The listing builds one solid part. Answer for the finished solid, in the listing's coordinates (mm). Give positions to 0.01 mm unless a question says otherwise; leave off trailing zeros. Write each loop counter-clockwise with the first axis right and the second up, starting at its lowest first coordinate (ties: lowest second). Pieces come first, ordered by that corner, then holes. Notation, with made-up numbers: (4.25, 54.25) -> (38.25, 54.25) arc R26 cw to (38.25, 81.25) -> close; hole circle Ø2 at (77.25, -2). An arc over 180 degrees is marked (long way). One line per question, with ' | ' between items.
from build123d import *

# Parameters (mm, degrees)
SKETCH_1_R      = 40
SKETCH_1_R_2    = 3.25
SKETCH_1_R_3    = 8.5
SKETCH_1_R_4    = 2.5
EXTRUDE_1_DEPTH = 4


with BuildPart() as part:
    # 草图1 → 凸台-拉伸1 (new body)
    with BuildSketch(Plane.XY):
        Circle(SKETCH_1_R)
        with Locations((0, 35)):
            Circle(SKETCH_1_R_2, mode=Mode.SUBTRACT)
        with Locations((30.310889132, 17.5)):
            Circle(SKETCH_1_R_2, mode=Mode.SUBTRACT)
        with Locations((30.310889132, -17.5)):
            Circle(SKETCH_1_R_2, mode=Mode.SUBTRACT)
        with Locations((0, -35)):
            Circle(SKETCH_1_R_2, mode=Mode.SUBTRACT)
        with Locations((-30.310889132, -17.5)):
            Circle(SKETCH_1_R_2, mode=Mode.SUBTRACT)
        with Locations((-30.310889132, 17.5)):
            Circle(SKETCH_1_R_2, mode=Mode.SUBTRACT)
        Circle(SKETCH_1_R_3, mode=Mode.SUBTRACT)
        with Locations((-9.25, 16.02146997)):
            Circle(SKETCH_1_R_4, mode=Mode.SUBTRACT)
        with Locations((16.02146997, 9.25)):
            Circle(SKETCH_1_R_4, mode=Mode.SUBTRACT)
        with Locations((9.25, -16.02146997)):
            Circle(SKETCH_1_R_4, mode=Mode.SUBTRACT)
        with Locations((-16.02146997, -9.25)):
            Circle(SKETCH_1_R_4, mode=Mode.SUBTRACT)
    extrude(amount=EXTRUDE_1_DEPTH)


solid = part.part
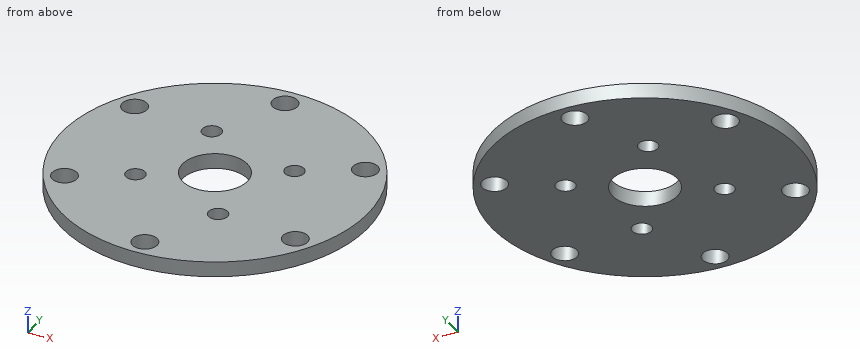
Item 1: Consider line 1 (Y direction, x = 0, z = 2.4); line 2 (Y direction, x = -30, z = 1.6); line 3 (Y direction, x = -2, z = 1.6). Determine where each line is inside the solid, lowest interval first. Write a range as [from, to].
Answers below:
line 1: [-40, -38.25], [-31.75, -8.5], [8.5, 31.75], [38.25, 40] | line 2: [-26.46, -20.74], [-14.26, 14.26], [20.74, 26.46] | line 3: [-39.95, -37.56], [-32.44, -8.26], [8.26, 32.44], [37.56, 39.95]
Item 2: Find section C-C (z = 2.9). Count the separate pieces of the cut face and the enclosed holes in it, then the cut area to 3 significant figures.
Answers below:
separate pieces: 1 | enclosed holes: 11 | area: 4,520 mm²
Item 3: Find section D-D (y = -24). Write down the section's boundary in (x, z), then the cut area to 3 significant figures.
Answers below:
outline: (-32, 0) -> (32, 0) -> (32, 4) -> (-32, 4) -> close | area: 256 mm²
Item 4: Find section A-A (y = 33). Write down the section's boundary in (x, z), then the cut area to 3 significant figures.
Answers below:
outline: (-22.61, 0) -> (-2.56, 0) -> (-2.56, 4) -> (-22.61, 4) -> close; (2.56, 0) -> (22.61, 0) -> (22.61, 4) -> (2.56, 4) -> close | area: 160 mm²
Item 5: Flat-ended cylindrical pins translate along their axes: pin 1 (5 mm diameter, centred on x = 0, y = -35, fed in from +Z); pin 2 (2 mm diameter, centred on x = -15.5, z = 3.5, fed in from +Y). Find the tip coordinate at first contact, or state that the pin passes through.
Answers below:
pin 1: through | pin 2: y = 37.28
Item 6: Find section B-B (y = 17.5). Write down the section's boundary in (x, z), then the cut area to 3 significant figures.
Answers below:
outline: (-35.97, 0) -> (-33.56, 0) -> (-33.56, 4) -> (-35.97, 4) -> close; (-27.06, 0) -> (-11.27, 0) -> (-11.27, 4) -> (-27.06, 4) -> close; (-7.23, 0) -> (27.06, 0) -> (27.06, 4) -> (-7.23, 4) -> close; (33.56, 0) -> (35.97, 0) -> (35.97, 4) -> (33.56, 4) -> close | area: 220 mm²
